from build123d import *


with BuildPart() as sphere:
    # Sphere → Sphere (revolve)
    with BuildSketch(Plane(origin=(0, 0, 71), x_dir=(1, 0, 0), z_dir=(0, -1, 0))):
        with BuildLine():
            ThreePointArc((0, -31), (31, 0), (0, 31))
            Line((0, 31), (0, -31))
        make_face()
    revolve(axis=Axis((0, 0, 71), (0, 0, 1)))


with BuildPart() as cut002:
    # Cone002 → Cone002 (revolve)
    with BuildSketch(Plane(origin=(0, 0, 49), x_dir=(1, 0, 0), z_dir=(0, -1, 0))):
        Polygon((0, 0), (29.5, 0), (31, 20), (0, 20), align=None)
    revolve(axis=Axis((0, 0, 49), (0, 0, 1)))

    # Cut002: cut Sphere
    add(sphere.part, mode=Mode.SUBTRACT)


with BuildPart() as part_mirroring002:
    # Part__Mirroring002: instance of Cut002
    add(cut002.part.mirror(Plane(origin=(0, 0, 0), x_dir=(0, -1, 0), z_dir=(1, 0, 0))))


solid = part_mirroring002.part
CAD build for the part. Positions are in the model's coordinates, mm. Round coordinates to 2 decimals unless told otherwise and drop trailing zeros. Order: outer loops, then holes, each group sorted by start corner. A loop starts at its lowest first (then second) coordinate and runs counter-clockwise, first axis right, second up. Notation, with made-up numbers: (5, 82) -> (34, 82) arc R36 cw to (34, 118) -> close; hole circle Ø5 at (2, 10). An arc over 180 degrees is marked (long way). Write item = value, one per line. Start each with the question number.
(1) Probe line 1 (X direction, y = -13, z = 61.5); line 2 (Y direction, x = 17.5, z = 58); line 3 (X direction, y = 6.5, z = 64.25). List the from-to ranges inside material, lowest first. Write a range as [from, to].
(2) Cut at A-A, the plane x = 0. List the corners of the cut face in (y, z), then the cut area to 3 significant figures.
(3) Cut at C-C, the plane z = 67.5. List the corners of the cut face in (x, y) (1 decimal).
(4) Pin check, flat tips, straight feed: P1, Ø1, axis at x = -22.5, z = 59, coming from the +Y side; P2, Ø1, axis at y = -11.5, z = 51, coming from the +X side; P3, Ø2, axis at x = 5.5, z = 57, coming from the +Y side. Stop position of each tip, or through.
(5) Cut at D-D, the plane z = 61.25. List the corners of the cut face in (x, y).
Model answer:
q1.line_1 = [-27.52, -26.49], [26.49, 27.52]
q1.line_2 = [-24.58, -22.04], [22.04, 24.58]
q1.line_3 = [-29.95, -29.55], [29.55, 29.95]
q2.outline = (-31, 69) -> (-29.5, 49) -> (-21.84, 49) arc R31 cw to (-30.94, 69) -> close; (21.84, 49) -> (29.5, 49) -> (31, 69) -> (30.94, 69) arc R31 cw to start
q2.area = 95.2 mm2
q3.outline = circle Ø61.8 at (0, 0); hole circle Ø61.6 at (0, 0)
q4.P1 = 20.76
q4.P2 = 27.54
q4.P3 = 29.78
q5.outline = circle Ø60.84 at (0, 0); hole circle Ø58.85 at (0, 0)
